Autodesk Inventor part; units mm, degrees
ref_plane "YZ Plane" through (0, 0, 0) normal (1, 0, 0) x (0, 1, 0)
ref_plane "XZ Plane" through (0, 0, 0) normal (0, 1, 0) x (-1, 0, 0)
ref_plane "XY Plane" through (0, 0, 0) normal (0, 0, 1) x (1, 0, 0)
sketch "tensioner_wood_block_base_sketch" plane through (0, 0, 0) normal (0, 1, 0) x (-1, 0, 0)
  line L0 (0, 0) -> (25.4, 0)
  line L1 (25.4, 0) -> (25.4, -63.5)
  line L2 (25.4, -63.5) -> (0, -63.5)
  line L3 (0, -63.5) -> (0, 0)
  dimension "d0" = 25.4
  dimension "d1" = 63.5
extrude "base_extrusion" add sketch "tensioner_wood_block_base_sketch" along normal blind 19.05
sketch "tensioner_sketch" plane through (-25.4, 0, -63.5) normal (-1, 0, 0) x (0, 0, 1)
  line L0 (41.275, 9.525) -> (22.225, 9.525) construction
  line L1 (41.275, 12.7) -> (22.225, 12.7)
  line L2 (22.225, 6.35) -> (41.275, 6.35)
  arc A0 (41.275, 6.35) -> (41.275, 12.7) centre (41.275, 9.525) ccw
  arc A1 (22.225, 12.7) -> (22.225, 6.35) centre (22.225, 9.525) ccw
  line L3 (63.5, 0) -> (63.5, 19.05)
  line L4 (63.5, 0) -> (0, 0)
  line L5 (31.75, 0) -> (31.75, 9.525) construction
  line L6 (31.75, 9.525) -> (31.75, 19.05) construction
  line L7 (0, 19.05) -> (63.5, 19.05)
  dimension "d4" = 22.225
  dimension "d5" = 19.05
  dimension "d6" = 6.35
extrude "tensioner" cut sketch "tensioner_sketch" against normal up to next
equation "\"d0\" = twb_width"
equation "\"d1\" = twb_height"
equation "\"d2\" = twb_length"
equation "\"d4\" = twb_tensioner_from_edge"
equation "\"d5\" = bp_tensioner_height"
equation "\"d6\" = bp_tensioner_width"
equation "\"d7\" = twb_length"
equation "\"bp_thickness\" = 3.048"
equation "\"bp_height\" = gb_mh_seperation + st_outer_diameter"
equation "\"bp_width\" = 6 * st_rivet_distance"
equation "\"bp_axle_height\" = magic_axle_offset + gb_axle_from_edge + gb_to_bottom_of_side_assembly"
equation "\"magic_axle_offset\" = 3.175"
equation "\"bp_tensioner_width\" = 6.35"
equation "\"bp_tensioner_height\" = 19.05"
equation "\"bp_tensioner_from_bottom\" = 50.8"
equation "\"bp_tensioner_from_side\" = 25.4"
equation "\"bp_tensioner_wood_mount_from_tensioner_top\" = 12.7"
equation "\"bp_tensioner_wood_mount_diameter\" = 6.35"
equation "\"gb_mh_seperation\" = 111.1504"
equation "\"gb_mh_diameter\" = 6.35"
equation "\"gb_axle_from_edge\" = 38.1"
equation "\"gb_width\" = 127"
equation "\"gb_bearing_diameter\" = 28.575"
equation "\"gb_to_bottom_of_side_assembly\" = 4.7752"
equation "\"rv_hole_diameter\" = 3.57187"
equation "\"st_outer_diameter\" = 25.4"
equation "\"st_wall_thickness\" = 6.35"
equation "\"st_length\" = 939.8"
equation "\"st_gbmh_from_center\" = 0.5 * gb_mh_seperation"
equation "\"st_cutout_depth_right\" = 342.9"
equation "\"st_cutout_depth_left\" = 342.9"
equation "\"st_rivet_distance\" = 19.05"
equation "\"so_inner_diameter\" = 6.35"
equation "\"so_wall_thickness\" = 3.048"
equation "\"so_length\" = 25.4"
equation "\"twb_width\" = st_outer_diameter"
equation "\"twb_length\" = bp_tensioner_width + 2 * twb_margin_on_each_side"
equation "\"twb_height\" = 2 * bp_tensioner_wood_mount_diameter + bp_tensioner_height + 2 * bp_tensioner_wood_mount_from_tensioner_top + twb_margin_on_each_side"
equation "\"twb_margin_on_each_side\" = 6.35"
equation "\"twb_tensioner_from_edge\" = -0.5 * bp_tensioner_height + 0.5 * twb_height"
properties part number "tensioner_wood_block(twb)" material "Wood (Oak)"
Could you check a few things on this model? Use its own coordinates, in mm. A direction names the side the tool comes from. Give positions to 0.01 mm unless a question says otherwise; leave off trailing zeros. Order: outer loops, then holes, each group sorted by start corner. A loop starts at its lowest first (then second) coordinate and runs counter-clockwise, first axis right, second up.
Item 1: If we section it at B-B, the plane y = 11.75: Write out the boundary of the cut face in (x, z).
Item 2: If we section it at C-C, the plane x = -18.25: Write out the boundary of the cut face in (y, z) (3 decimals).
Item 3: If we mould it in two halves opening along Y, with no side actions, what happens to faces 3 (the face through (-13, 12.7, -32)), 4 (the face through (-25.4, 14, -31)), 5 (the face through (-13, 19.05, -31))? For each: pulls with the +Y half, pulls with the -Y half, needs draft (parallel to the pull), parting line crosses it, or undercut.
Item 4: I need wall thicknesses on line 1 (Y direction, x = -21.25, z = -24.5); line 2 (Z direction, x = -22.5, y = 9.5); line 3 (Z direction, x = -18, y = 7.25). Which ranges of each line are inside material? Lowest first, please.
Item 5: If we section it at A-A, the plane z = -32.5: Write out the boundary of the cut face in (x, y).
Item 6: For faces 1 (the face through (-13, 0, -31)), 2 (the face through (-12.88, 9.46, -19.05)), which set-ups out of +Z, -Z, +X, -X, +Y, -Y let a thin tool reach every point of the face, with its end or its side?
Values:
1. outline: (-25.4, -63.5) - (0, -63.5) - (0, -43.54) - (-25.4, -43.54) - close; (-25.4, -19.96) - (0, -19.96) - (0, 0) - (-25.4, 0) - close
2. outline: (0, -63.5) - (19.05, -63.5) - (19.05, 0) - (0, 0) - close; hole (6.35, -41.275) arc R3.175 ccw to (12.7, -41.275) - (12.7, -22.225) arc R3.175 ccw to (6.35, -22.225) - close
3. face 3: undercut
3. face 4: needs draft
3. face 5: pulls with the +Y half
4. line 1: y = 0 to 6.35, 12.7 to 19.05
4. line 2: z = -63.5 to -44.45, -19.05 to 0
4. line 3: z = -63.5 to -43.49, -20.01 to 0
5. outline: (-25.4, 0) - (0, 0) - (0, 6.35) - (-25.4, 6.35) - close; (-25.4, 12.7) - (0, 12.7) - (0, 19.05) - (-25.4, 19.05) - close
6. face 1: +Z, -Z, +X, -X, -Y
6. face 2: +X, -X
